```python
from build123d import *

# Parameters (mm, degrees)
CHAMFER1_SIZE      = 0.79375
CUT_EXTRUDE1_DEPTH = 34.294897541
CHAMFER2_SIZE      = 0.79375


with BuildPart() as part:
    # Sketch1 → Revolve1 (revolve)
    with BuildSketch(Plane.XY, mode=Mode.PRIVATE) as revolve1_sk:
        with BuildLine():
            Line((0, 0), (15.1765, 0))
            Line((15.1765, 0), (15.1765, 20.955))
            Line((15.1765, 20.955), (10.414, 20.955))
            Line((10.414, 20.955), (10.414, 16.1925))
            ThreePointArc((10.414, 16.1925), (6.985, 12.7635), (3.556, 16.1925))
            Line((3.556, 16.1925), (3.556, 20.955))
            Line((3.556, 20.955), (0, 20.955))
            Line((0, 20.955), (0, 0))
        make_face()
    revolve(revolve1_sk.sketch.rotate(Axis((0, 0, 0), (1, 0, 0)), 90), axis=Axis((0, 0, 0), (1, 0, 0)))

    # Chamfer1
    chamfer1_edges = [part.edges().sort_by_distance(p)[0] for p in [
        (0, 0, -20.955),
    ]]
    chamfer(chamfer1_edges, length=CHAMFER1_SIZE)

    # Sketch2 → Cut-Extrude1 (cut, through all)
    with BuildSketch(Plane.ZY):
        Polygon((3.673506558, -6.3627), (7.347013116, 0), (3.673506558, 6.3627), (-3.673506558, 6.3627), (-7.347013116, 0), (-3.673506558, -6.3627), align=None)
    extrude(amount=-CUT_EXTRUDE1_DEPTH, mode=Mode.SUBTRACT)

    # Chamfer2
    chamfer2_edges = [part.edges().sort_by_distance(p)[0] for p in [
        (3.556, 0, -20.955),
        (10.414, 0, -20.955),
        (15.1765, 0, -20.955),
    ]]
    chamfer(chamfer2_edges, length=CHAMFER2_SIZE)


solid = part.part
```
The listing builds one solid part. Answer for the finished solid, in the listing's coordinates (mm). A direction names the side the tool comes from. Coordinates: 2 decimals unless noted, no trailing zeros. Loops run counter-clockwise (first coordinate to the right, second up) from the corner with the lowest first, then second, coordinate; pieces in that order, holes last. Notation, with made-up numbers: (15.5, 21.25) - (41.5, 21.25) arc R32 cw to (41.5, 60.25) - close; hole circle Ø1 at (52.25, -2). An arc over 180 degrees is marked (long way). Use a Markdown table: item, result. Add a question column.
1) The mould has two halves that part along X. Classify faces 3 (the flat face through (10.414, -17, 0)), 4 (the flat face through (7.5, 3.2, -5.5)), 5 (the flat face through (0, -5, -5)), 6 (the flat face through (15.176, -5, 5)): released by +X, released by -X, zero draft, split by the parting line, or undercut.
2) The part is cut by section B-B, the plane x = 7.25. Give the vertices of the cut face in (y, z).
3) Find the intervals of material crossed by line 1 (X direction, y = 6, z = -17); line 2 (Y direction, x = 9.75, z = -1.5); line 3 (Y direction, x = 12, z = 3), in increasing order.
4) For faces 1 (the flat face through (7.482, -3.137, -5.536)), 2 (the flat face through (3.556, -17, 0)), determine the directions among +Z, -Z, +X, -X, +Y, -Y from which every point of the face is accessible in a straight line to the end or side of a thin tool.
5) Given pin 1 (6 mm diameter, centred on x = 8, y = -14.5, fed in from -Z); pin 2 (1 mm diameter, centred on x = 13.5, y = 10, fed in from -Z); pin 3 (3 mm diameter, centred on y = 7, z = 2, fed in from -X); pin 4 (6 mm diameter, centred on x = 13, z = -10.5, fed in from +Y), each flat-ended and moving along its own axis, determine where each tip first touches the part or whether it passes through.
6) The part is cut by section A-A, the plane z = 0. Give the vertices of the cut face in (x, y) (1 decimal).
Here are the results:
| question | item | result |
|---|---|---|
| 1 | face 3 | undercut |
| 1 | face 4 | zero draft |
| 1 | face 5 | released by -X |
| 1 | face 6 | released by +X |
| 2 | outline | circle Ø25.55 at (0, 0); hole (-6.36, -3.67) - (0, -7.35) - (6.36, -3.67) - (6.36, 3.67) - (0, 7.35) - (-6.36, 3.67) - close |
| 3 | line 1 | x = 0 to 3.56, 10.41 to 15.18 |
| 3 | line 2 | y = -14.08 to -6.36, 6.36 to 14.08 |
| 3 | line 3 | y = -20.74 to -6.36, 6.36 to 20.74 |
| 4 | face 1 | +X, -X |
| 4 | face 2 | none |
| 5 | pin 1 | stops at z = -15.65 |
| 5 | pin 2 | stops at z = -18.68 |
| 5 | pin 3 | stops at x = 0 |
| 5 | pin 4 | stops at y = 19.57 |
| 6 | outline | (0, -20.2) - (0.8, -21) - (2.8, -21) - (3.6, -20.2) - (3.6, -16.2) arc R3.4 cw to (10.4, -16.2) - (10.4, -20.2) - (11.2, -21) - (14.4, -21) - (15.2, -20.2) - (15.2, -6.4) - (0, -6.4) - close; (0, 6.4) - (15.2, 6.4) - (15.2, 20.2) - (14.4, 21) - (11.2, 21) - (10.4, 20.2) - (10.4, 16.2) arc R3.4 cw to (3.6, 16.2) - (3.6, 20.2) - (2.8, 21) - (0.8, 21) - (0, 20.2) - close |
